```python
from build123d import *

# Parameters (mm, degrees)
ESQUISSE1_R      = 1.6
EXTRUSION1_DEPTH = 2
ESQUISSE2_W      = 29.5
ESQUISSE2_H      = 13
EXTRUSION2_DEPTH = 11.5
ESQUISSE3_W      = 10
ESQUISSE3_H      = 5
EXTRUSION3_DEPTH = 6


with BuildPart() as part:
    # Esquisse1 → Extrusion1 (new body)
    with BuildSketch(Plane.XY):
        with BuildLine():
            Line((-18.5, -6.5), (18.5, -6.5))
            ThreePointArc((18.5, -6.5), (25, 0), (18.5, 6.5))
            Line((18.5, 6.5), (-18.5, 6.5))
            ThreePointArc((-18.5, 6.5), (-25, 0), (-18.5, -6.5))
        make_face()
        with Locations((-18.5, 0)):
            Circle(ESQUISSE1_R, mode=Mode.SUBTRACT)
        with Locations((18.5, 0)):
            Circle(ESQUISSE1_R, mode=Mode.SUBTRACT)
    extrude(amount=EXTRUSION1_DEPTH)

    # Esquisse2 → Extrusion2 (add)
    with BuildSketch(Plane.XY.offset(2)):
        Rectangle(ESQUISSE2_W, ESQUISSE2_H)
    extrude(amount=EXTRUSION2_DEPTH)

    # Esquisse3 → Extrusion3 (add)
    with BuildSketch(Plane.XZ.offset(6.5)):
        with Locations((0, 5.8)):
            Rectangle(ESQUISSE3_W, ESQUISSE3_H)
    extrude(amount=EXTRUSION3_DEPTH)


solid = part.part
```
Geometry check sheet. Reference: the model listing, model coordinates, mm. A direction names the side the tool comes from. Give positions to 0.01 mm unless a question says otherwise; leave off trailing zeros. Loops run counter-clockwise (first coordinate to the right, second up) from the corner with the lowest first, then second, coordinate; pieces in that order, holes last. Notation, with made-up numbers: M 1.5,0 L 53.5,0 A24 cw 53.5,26 Z; hole C 51.5,-7.75 d6. An arc over 180 degrees is marked long. Write item = value, one per line.
(1) Sectioned sample at C-C, the plane x = -18. Record the cut outline in (y, z), plus the area to 3 significant figures.
Answer below:
outline = M -6.5,0 L -1.52,0 L -1.52,2 L -6.5,2 Z; M 1.52,0 L 6.5,0 L 6.5,2 L 1.52,2 Z
area = 19.9 mm2
(2) Sectioned sample at D-D, the plane z = 5. Record the cut outline in (x, y).
Answer below:
outline = M -14.75,-6.5 L -5,-6.5 L -5,-12.5 L 5,-12.5 L 5,-6.5 L 14.75,-6.5 L 14.75,6.5 L -14.75,6.5 Z
(3) Sectioned sample at B-B, the plane x = -2. Record the cut outline in (y, z).
Answer below:
outline = M -12.5,3.3 L -6.5,3.3 L -6.5,0 L 6.5,0 L 6.5,13.5 L -6.5,13.5 L -6.5,8.3 L -12.5,8.3 Z
(4) Gauge pin test, flat ends, axial feed: pin 1 Ø3 at (x, y) = (1, -9.5) entering from -Z; pin 2 Ø8 at (x, y) = (-21, 1) entering from +Z; pin 3 Ø1 at (x, y) = (-7, -8.5) entering from +Z; pin 4 Ø3.5 at (y, z) = (0.5, 9) entering from -X. Record the tip position at first contact, or that the pin passes through.
Answer below:
pin_1 = 3.3
pin_2 = 2
pin_3 = through
pin_4 = -14.75
(5) Tool access check on faces 5 (the face through (0, -9, 3.3)), 6 (the face through (5, -9, 6)), 7 (the face through (-20, -1, 2)), 8 (the face through (20, -1, 2)). Record the directions out of +Z, -Z, +X, -X, +Y, -Y that give a thin tool (end or side, any length) a straight path to the whole face; none if there is none.
Answer below:
face_5 = -Z, +X, -X, -Y
face_6 = +Z, -Z, +X, -Y
face_7 = +Z, -X, +Y, -Y
face_8 = +Z, +X, +Y, -Y
(6) Release check for a two-part mould opening along X. For faces 1 (the face through (-20.1, 0.07, 0.99)), 2 (the face through (0, 0, 0)), 3 (the face through (17.32, 1.08, 0.99)), 4 (the face through (-25, 0, 1)) record: released by +X, released by -X, zero draft, split by the parting line, or undercut.
Answer below:
face_1 = undercut
face_2 = zero draft
face_3 = undercut
face_4 = released by -X
(7) Sectioned sample at A-A, the plane y = 0. Record the cut outline in (x, z).
Answer below:
outline = M -25,0 L -20.1,0 L -20.1,2 L -25,2 Z; M -16.9,0 L 16.9,0 L 16.9,2 L 14.75,2 L 14.75,13.5 L -14.75,13.5 L -14.75,2 L -16.9,2 Z; M 20.1,0 L 25,0 L 25,2 L 20.1,2 Z
(8) Material ranges on line 1 (Y direction, x = -18.5, z = 1.4); line 2 (Y direction, x = 5.5, z = 4); line 3 (Z direction, x = -20.5, y = 5), recorded low to high. Write a range as [from, to].
Answer below:
line_1 = [-6.5, -1.6], [1.6, 6.5]
line_2 = [-6.5, 6.5]
line_3 = [0, 2]
